```python
from build123d import *

# Parameters (mm, degrees)
F0_R     = 13.5
F0_R_2   = 11.5
F1_DEPTH = 15
F0_W     = 36
F0_H     = 36
F0_R_3   = 1.75
F2_DEPTH = 3
F3_R     = 5


with BuildPart() as f1:
    # F0 (on Front) → F1 (new body)
    with BuildSketch(Plane.XZ):
        Circle(F0_R)
        Circle(F0_R_2, mode=Mode.SUBTRACT)
    extrude(amount=F1_DEPTH)

    # F0 (on Front) → F2 (join)
    with BuildSketch(Plane.XZ):
        Rectangle(F0_W, F0_H)
        with Locations((-14.142136, -14.142136)):
            Circle(F0_R_3, mode=Mode.SUBTRACT)
        with Locations((14.142136, -14.142136)):
            Circle(F0_R_3, mode=Mode.SUBTRACT)
        with Locations((-14.142136, 14.142136)):
            Circle(F0_R_3, mode=Mode.SUBTRACT)
        Circle(F0_R, mode=Mode.SUBTRACT)
        with Locations((14.142136, 14.142136)):
            Circle(F0_R_3, mode=Mode.SUBTRACT)
    extrude(amount=F2_DEPTH)

    # F3
    f3_edges = [f1.edges().sort_by_distance(p)[0] for p in [
        (18, -1.5, -18),
        (18, -1.5, 18),
        (-18, -1.5, 18),
        (-18, -1.5, -18),
    ]]
    fillet(f3_edges, radius=F3_R)


solid = f1.part
```
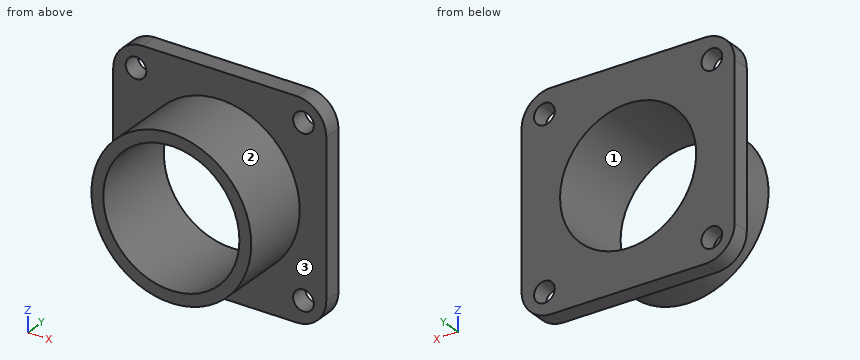
Check sheet for the modelled part. Datum: model origin and axes. Units: mm. Face numbers are marked on the shaded views. Round coordinates to 2 decimals unless told otherwise and drop trailing zeros. Write each loop counter-clockwise with the first axis right and the second up, starting at its lowest first coordinate (ties: lowest second). Pieces come first, ordered by that corner, then holes. Notation, with made-up numbers: (85.25, 39) -> (142.25, 39) arc R35 cw to (142.25, 77) -> close; hole circle Ø10 at (60.5, -25). An arc over 180 degrees is marked (long way). Put each result on its own line as item: value.
(1) Mould release check, pull along Z, two halves, no side actions. Record for the marked faces 1, 2 and 3: released by +Z, released by -Z, zero draft, split by the parting line, or undercut.
Values found:
face 1: undercut
face 2: split by the parting line
face 3: zero draft
(2) Sectioned sample at A-A (z = 0). Enter the section's corners in (x, y), plus the area to 3 significant figures.
Values found:
outline: (-18, -3) -> (-13.5, -3) -> (-13.5, -15) -> (-11.5, -15) -> (-11.5, 0) -> (-18, 0) -> close; (11.5, -15) -> (13.5, -15) -> (13.5, -3) -> (18, -3) -> (18, 0) -> (11.5, 0) -> close
area: 87.0 mm^2
(3) Go/stop test with flat-tipped pins: pin 1 Ø4 at (x, z) = (-14.14, -14.14) entering from +Y; pin 2 Ø4 at (y, z) = (-10, -1.5) entering from -X; pin 3 Ø4 at (y, z) = (-9, -12) entering from +X; pin 4 Ø5 at (x, y) = (-1, -6) entering from +Z. Record where each tip stops, or that it passes through.
Values found:
pin 1: stops at y = 0
pin 2: stops at x = -13.5
pin 3: stops at x = 9.07
pin 4: stops at z = 13.5
(4) Sectioned sample at D-D (x = -14.5). Enter the section's corners in (y, z), plus the area to 3 significant figures.
Values found:
outline: (-3, -17.77) -> (0, -17.77) -> (0, -15.86) -> (-3, -15.86) -> close; (-3, -12.43) -> (0, -12.43) -> (0, 12.43) -> (-3, 12.43) -> close; (-3, 15.86) -> (0, 15.86) -> (0, 17.77) -> (-3, 17.77) -> close
area: 86.1 mm^2
(5) Sectioned sample at B-B (x = 0). Enter the section's corners in (y, z).
Values found:
outline: (-15, -13.5) -> (-3, -13.5) -> (-3, -18) -> (0, -18) -> (0, -11.5) -> (-15, -11.5) -> close; (-15, 11.5) -> (0, 11.5) -> (0, 18) -> (-3, 18) -> (-3, 13.5) -> (-15, 13.5) -> close
(6) Sectioned sample at C-C (z = -15). Enter the section's corners in (x, y).
Values found:
outline: (-17.58, -3) -> (-15.67, -3) -> (-15.67, 0) -> (-17.58, 0) -> close; (-12.62, -3) -> (12.62, -3) -> (12.62, 0) -> (-12.62, 0) -> close; (15.67, -3) -> (17.58, -3) -> (17.58, 0) -> (15.67, 0) -> close
(7) Material ranges on line 1 (Z direction, x = 9.5, y = -4.5); line 2 (Z direction, x = -5.5, y = -8.75); line 3 (X direction, y = -14, z = -10), recorded low to high.
Values found:
line 1: z = -9.59 to -6.48, 6.48 to 9.59
line 2: z = -12.33 to -10.1, 10.1 to 12.33
line 3: x = -9.07 to -5.68, 5.68 to 9.07
